Geometry: final body of the model. Coordinates: model frame, mm. Give positions to 0.01 mm unless a question says otherwise; leave off trailing zeros. Write each loop counter-clockwise with the first axis right and the second up, starting at its lowest first coordinate (ties: lowest second). Pieces come first, ordered by that corner, then holes. Notation, with made-up numbers: (17, 21.25) - (29, 21.25) arc R24 ccw to (29, 49.25) - close; hole circle Ø1 at (43, -33). An arc over 180 degrees is marked (long way). Return JSON: item names as keys, results as strings.
from build123d import *

# Parameters (mm, degrees)
BOSS_EXTRUDE1_DEPTH            = 2.5
M5_CLEARANCE_HOLE1_D           = 5.5
M5_CLEARANCE_HOLE1_CSINK_D     = 5.55
M5_CLEARANCE_HOLE1_CSINK_ANGLE = 90


with BuildPart() as part:
    # Sketch1 → Boss-Extrude1 (new, symmetric)
    with BuildSketch(Plane(origin=(0, 0, 0), x_dir=(1, 0, 0), z_dir=(0, 1, 0))):
        Polygon((45, 15), (40, 15), (35, 15), (35, 10), (25, 10), (25, 15), (15, 15), (15, 10), (5, 10), (5, 15), (-5, 15), (-5, 10), (-15, 10), (-15, 15), (-25, 15), (-25, 10), (-35, 10), (-35, 15), (-40, 15), (-45, 15), (-45, 10), (-45, 5), (-40, 5), (-40, -5), (-45, -5), (-45, -10), (-45, -15), (-40, -15), (-35, -15), (-35, -10), (-25, -10), (-25, -15), (-15, -15), (-15, -10), (-5, -10), (-5, -15), (5, -15), (5, -10), (15, -10), (15, -15), (25, -15), (25, -10), (35, -10), (35, -15), (40, -15), (45, -15), (45, -10), (45, -5), (40, -5), (40, 5), (45, 5), (45, 10), align=None)
    extrude(amount=BOSS_EXTRUDE1_DEPTH, both=True)

    # M5 Clearance Hole1 (through all)
    with Locations(Plane(origin=(0, 2.5, 0), x_dir=(1, 0, 0), z_dir=(0, 1, 0))):
        with Locations((12.5, 4.5), (-12.5, 4.5)):
            CounterSinkHole(M5_CLEARANCE_HOLE1_D / 2, M5_CLEARANCE_HOLE1_CSINK_D / 2, counter_sink_angle=M5_CLEARANCE_HOLE1_CSINK_ANGLE)


solid = part.part
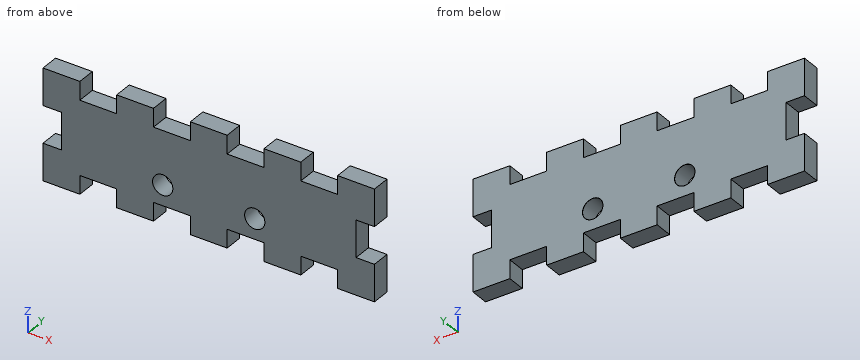
Q1. Section query B-B, the plane z = 11.25. Return the cut outline in (x, y), plus the area to 3 significant figures.
Answer key:
{"outline": "(-45, -2.5) - (-35, -2.5) - (-35, 2.5) - (-45, 2.5) - close; (-25, -2.5) - (-15, -2.5) - (-15, 2.5) - (-25, 2.5) - close; (-5, -2.5) - (5, -2.5) - (5, 2.5) - (-5, 2.5) - close; (15, -2.5) - (25, -2.5) - (25, 2.5) - (15, 2.5) - close; (35, -2.5) - (45, -2.5) - (45, 2.5) - (35, 2.5) - close", "area": "250 mm^2"}
Q2. Section query D-D, the plane z = 1. Return the cut outline in (x, y).
Answer key:
{"outline": "(-40, -2.5) - (40, -2.5) - (40, 2.5) - (-40, 2.5) - close"}
Q3. Section query A-A, the plane x = -12.5. Return the cut outline in (y, z) (3 decimals), plus the area to 3 significant figures.
Answer key:
{"outline": "(-2.5, -10) - (2.5, -10) - (2.5, -7.275) - (2.475, -7.25) - (-2.5, -7.25) - close; (-2.5, -1.75) - (2.475, -1.75) - (2.5, -1.725) - (2.5, 10) - (-2.5, 10) - close", "area": "72.5 mm^2"}
Q4. Section query C-C, the plane y = 0.9. Count the separate pieces of the cut face and the enclosed holes in it, plus the area to 3 significant figures.
Answer key:
{"separate pieces": "1", "enclosed holes": "2", "area": "2,150 mm^2"}
Q5. Material intervals for probe 1 along X at (y, z) = (2.1, -10.5); probe 2 along X at (y, z) = (-0.65, -2.25); probe 3 along Z at (x, y) = (-12.5, 1.15), sorted ascending. Write a range as [from, to].
Answer key:
{"probe 1": "x = [-45, -35], [-25, -15], [-5, 5], [15, 25], [35, 45]", "probe 2": "x = [-40, -14.08], [-10.92, 10.92], [14.08, 40]", "probe 3": "z = [-10, -7.25], [-1.75, 10]"}
Q6. Pin query (flat end, axial travel): P1, Ø2, axis at x = -8, y = -1, coming from the -Z side; P2, Ø1.5, axis at x = 30.5, y = -1, coming from the +Z side. Return the tip coordinate at first contact, or that it passes through.
Answer key:
{"P1": "stops at z = -10", "P2": "stops at z = 10"}
